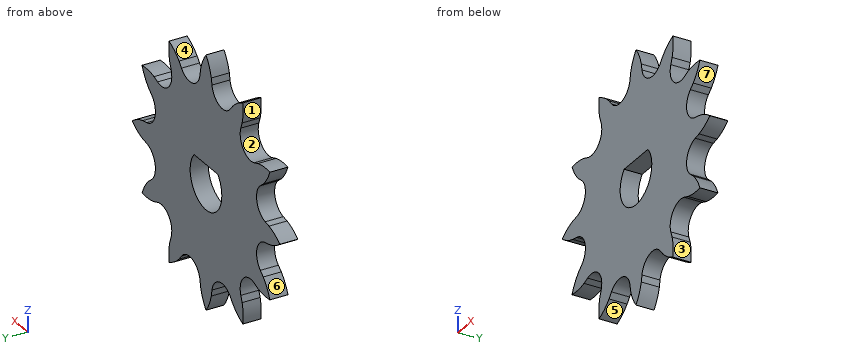
from build123d import *

# Parameters (mm, degrees)
SKETCH1_R           = 10
BOSS_EXTRUDE3_DEPTH = 2
CUT_EXTRUDE4_START  = -2
CUT_EXTRUDE4_DEPTH  = 2
CUT_EXTRUDE5_DEPTH  = 2
CUT_EXTRUDE7_START  = -2
CUT_EXTRUDE7_DEPTH  = 2


with BuildPart() as part:
    # Sketch1 → Boss-Extrude3 (new body)
    # profile 1 of 3: a face of its own
    with BuildSketch(Plane(origin=(0, 0, 0), x_dir=(1, 0, 0), z_dir=(0, 1, 0))):
        with BuildLine():
            ThreePointArc((-2.576546391, 9.66237076), (-3.696714803, 9.688501423), (-4.6270391, 10.312966622))
            Line((-4.6270391, 10.312966622), (-5.089759275, 10.867122458))
            add(Edge.make_bspline(
                [(-5.089759275, 10.867122458), (-6.64901802, 12.325915574), (-6.970753087, 12.141194398)],
                knots=[0, 0, 0, 1, 1, 1], degree=2, weights=[1, 1.687053572, 1]))
            ThreePointArc((-6.970753087, 12.141194398), (-7.014608214, -12.115909855), (14, 0))
            ThreePointArc((14, 0), (9.899494937, 9.899494937), (0, 14))
            add(Edge.make_bspline(
                [(-0.996876474, 11.958521535), (-0.370992408, 14), (0, 14)],
                knots=[0, 0, 0, 1, 1, 1], degree=2, weights=[1, 1.687053572, 1]))
            Line((-0.996876474, 11.958521535), (-1.122240194, 11.247548548))
            ThreePointArc((-1.122240194, 11.247548548), (-1.618115564, 10.242776114), (-2.576546391, 9.66237076))
        make_face()
        with BuildLine():
            ThreePointArc((10, 0), (-6.092394278, -7.9298633), (-2.576546391, 9.66237076))
            ThreePointArc((-2.576546391, 9.66237076), (6.092394278, 7.9298633), (10, 0))
        make_face(mode=Mode.SUBTRACT)
    # profile 2 of 3: a face of its own
    with BuildSketch(Plane(origin=(0, 0, 0), x_dir=(1, 0, 0), z_dir=(0, 1, 0))):
        Circle(SKETCH1_R)
    # profile 3 of 3: a face of its own
    with BuildSketch(Plane(origin=(0, 0, 0), x_dir=(1, 0, 0), z_dir=(0, 1, 0))):
        with BuildLine():
            Line((-5.089759275, 10.867122458), (-4.6270391, 10.312966622))
            ThreePointArc((-4.6270391, 10.312966622), (-3.696714803, 9.688501423), (-2.576546391, 9.66237076))
            ThreePointArc((-2.576546391, 9.66237076), (-1.618115564, 10.242776114), (-1.122240194, 11.247548548))
            Line((-1.122240194, 11.247548548), (-0.996876474, 11.958521535))
            add(Edge.make_bspline(
                [(-0.996876474, 11.958521535), (-0.370992408, 14), (0, 14)],
                knots=[0, 0, 0, 1, 1, 1], degree=2, weights=[1, 1.687053572, 1]))
            ThreePointArc((0, 14), (-3.607164983, 13.527319054), (-6.970753087, 12.141194398))
            add(Edge.make_bspline(
                [(-5.089759275, 10.867122458), (-6.64901802, 12.325915574), (-6.970753087, 12.141194398)],
                knots=[0, 0, 0, 1, 1, 1], degree=2, weights=[1, 1.687053572, 1]))
        make_face()
    extrude(amount=BOSS_EXTRUDE3_DEPTH)

    # Sketch2 → Cut-Extrude4 (cut)
    with BuildSketch(Plane(origin=(0, 2, 0), x_dir=(1, 0, 0), z_dir=(0, 1, 0)).offset(CUT_EXTRUDE4_START)):
        with BuildLine():
            Line((-1.136213035, 11.24381356), (-1.010390736, 11.95738728))
            ThreePointArc((-1.010390736, 11.95738728), (-0.613638742, 13.032335811), (0, 14))
            ThreePointArc((0, 14), (-3.623466631, 13.522961568), (-7, 12.124355653))
            ThreePointArc((-7, 12.124355653), (-5.984741166, 11.593153253), (-5.103669595, 10.860596515))
            Line((-5.103669595, 10.860596515), (-4.637917427, 10.305534696))
            ThreePointArc((-4.637917427, 10.305534696), (-2.588190451, 9.659258263), (-1.136213035, 11.24381356))
        make_face()
    extrude(amount=CUT_EXTRUDE4_DEPTH, mode=Mode.SUBTRACT)

    # Sketch3 → Cut-Extrude5 (cut)
    with BuildSketch(Plane(origin=(0, 2, 0), x_dir=(1, 0, 0), z_dir=(0, 1, 0))):
        with BuildLine():
            Line((-2.25, -1.984313483), (2.25, -1.984313483))
            ThreePointArc((2.25, -1.984313483), (0, 3), (-2.25, -1.984313483))
        make_face()
    extrude(amount=-CUT_EXTRUDE5_DEPTH, mode=Mode.SUBTRACT)

    # Sketch2<5> → Cut-Extrude7 (cut)
    with BuildSketch(Plane(origin=(0, 2, 0), x_dir=(1, 0, 0), z_dir=(0, 1, 0)).offset(CUT_EXTRUDE7_START)):
        with BuildLine():
            ThreePointArc((7, 12.124355653), (3.623466631, 13.522961568), (0, 14))
            ThreePointArc((0, 14), (0.613638742, 13.032335811), (1.010390736, 11.95738728))
            Line((1.010390736, 11.95738728), (1.136213035, 11.24381356))
            ThreePointArc((1.136213035, 11.24381356), (2.588190451, 9.659258263), (4.637917427, 10.305534696))
            Line((4.637917427, 10.305534696), (5.103669595, 10.860596515))
            ThreePointArc((5.103669595, 10.860596515), (5.984741166, 11.593153253), (7, 12.124355653))
        make_face()
        with BuildLine():
            ThreePointArc((12.124355653, 7), (9.899494937, 9.899494937), (7, 12.124355653))
            ThreePointArc((7, 12.124355653), (7.047594644, 10.979514512), (6.853717685, 9.850205779))
            Line((6.853717685, 9.850205779), (6.605896133, 9.169321661))
            ThreePointArc((6.605896133, 9.169321661), (7.071067812, 7.071067812), (9.169321661, 6.605896133))
            Line((9.169321661, 6.605896133), (9.850205779, 6.853717685))
            ThreePointArc((9.850205779, 6.853717685), (10.979514512, 7.047594644), (12.124355653, 7))
        make_face()
        with BuildLine():
            ThreePointArc((14, 0), (13.522961568, 3.623466631), (12.124355653, 7))
            ThreePointArc((12.124355653, 7), (11.593153253, 5.984741166), (10.860596515, 5.103669595))
            Line((10.860596515, 5.103669595), (10.305534696, 4.637917427))
            ThreePointArc((10.305534696, 4.637917427), (9.659258263, 2.588190451), (11.24381356, 1.136213035))
            Line((11.24381356, 1.136213035), (11.95738728, 1.010390736))
            ThreePointArc((11.95738728, 1.010390736), (13.032335811, 0.613638742), (14, 0))
        make_face()
        with BuildLine():
            ThreePointArc((-6.853717685, 9.850205779), (-7.047594644, 10.979514512), (-7, 12.124355653))
            ThreePointArc((-7, 12.124355653), (-9.899494937, 9.899494937), (-12.124355653, 7))
            ThreePointArc((-12.124355653, 7), (-10.979514512, 7.047594644), (-9.850205779, 6.853717685))
            Line((-9.850205779, 6.853717685), (-9.169321661, 6.605896133))
            ThreePointArc((-9.169321661, 6.605896133), (-7.071067812, 7.071067812), (-6.605896133, 9.169321661))
            Line((-6.605896133, 9.169321661), (-6.853717685, 9.850205779))
        make_face()
        with BuildLine():
            ThreePointArc((12.124355653, -7), (13.522961568, -3.623466631), (14, 0))
            ThreePointArc((14, 0), (13.032335811, -0.613638742), (11.95738728, -1.010390736))
            Line((11.95738728, -1.010390736), (11.24381356, -1.136213035))
            ThreePointArc((11.24381356, -1.136213035), (9.659258263, -2.588190451), (10.305534696, -4.637917427))
            Line((10.305534696, -4.637917427), (10.860596515, -5.103669595))
            ThreePointArc((10.860596515, -5.103669595), (11.593153253, -5.984741166), (12.124355653, -7))
        make_face()
        with BuildLine():
            ThreePointArc((-10.860596515, 5.103669595), (-11.593153253, 5.984741166), (-12.124355653, 7))
            ThreePointArc((-12.124355653, 7), (-13.522961568, 3.623466631), (-14, 0))
            ThreePointArc((-14, 0), (-13.032335811, 0.613638742), (-11.95738728, 1.010390736))
            Line((-11.95738728, 1.010390736), (-11.24381356, 1.136213035))
            ThreePointArc((-11.24381356, 1.136213035), (-9.659258263, 2.588190451), (-10.305534696, 4.637917427))
            Line((-10.305534696, 4.637917427), (-10.860596515, 5.103669595))
        make_face()
        with BuildLine():
            ThreePointArc((7, -12.124355653), (9.899494937, -9.899494937), (12.124355653, -7))
            ThreePointArc((12.124355653, -7), (10.979514512, -7.047594644), (9.850205779, -6.853717685))
            Line((9.850205779, -6.853717685), (9.169321661, -6.605896133))
            ThreePointArc((9.169321661, -6.605896133), (7.071067812, -7.071067812), (6.605896133, -9.169321661))
            Line((6.605896133, -9.169321661), (6.853717685, -9.850205779))
            ThreePointArc((6.853717685, -9.850205779), (7.047594644, -10.979514512), (7, -12.124355653))
        make_face()
        with BuildLine():
            ThreePointArc((-11.95738728, -1.010390736), (-13.032335811, -0.613638742), (-14, 0))
            ThreePointArc((-14, 0), (-13.522961568, -3.623466631), (-12.124355653, -7))
            ThreePointArc((-12.124355653, -7), (-11.593153253, -5.984741166), (-10.860596515, -5.103669595))
            Line((-10.860596515, -5.103669595), (-10.305534696, -4.637917427))
            ThreePointArc((-10.305534696, -4.637917427), (-9.659258263, -2.588190451), (-11.24381356, -1.136213035))
            Line((-11.24381356, -1.136213035), (-11.95738728, -1.010390736))
        make_face()
        with BuildLine():
            ThreePointArc((0, -14), (3.623466631, -13.522961568), (7, -12.124355653))
            ThreePointArc((7, -12.124355653), (5.984741166, -11.593153253), (5.103669595, -10.860596515))
            Line((5.103669595, -10.860596515), (4.637917427, -10.305534696))
            ThreePointArc((4.637917427, -10.305534696), (2.588190451, -9.659258263), (1.136213035, -11.24381356))
            Line((1.136213035, -11.24381356), (1.010390736, -11.95738728))
            ThreePointArc((1.010390736, -11.95738728), (0.613638742, -13.032335811), (0, -14))
        make_face()
        with BuildLine():
            ThreePointArc((-9.850205779, -6.853717685), (-10.979514512, -7.047594644), (-12.124355653, -7))
            ThreePointArc((-12.124355653, -7), (-9.899494937, -9.899494937), (-7, -12.124355653))
            ThreePointArc((-7, -12.124355653), (-7.047594644, -10.979514512), (-6.853717685, -9.850205779))
            Line((-6.853717685, -9.850205779), (-6.605896133, -9.169321661))
            ThreePointArc((-6.605896133, -9.169321661), (-7.071067812, -7.071067812), (-9.169321661, -6.605896133))
            Line((-9.169321661, -6.605896133), (-9.850205779, -6.853717685))
        make_face()
        with BuildLine():
            ThreePointArc((-7, -12.124355653), (-3.623466631, -13.522961568), (0, -14))
            ThreePointArc((0, -14), (-0.613638742, -13.032335811), (-1.010390736, -11.95738728))
            Line((-1.010390736, -11.95738728), (-1.136213035, -11.24381356))
            ThreePointArc((-1.136213035, -11.24381356), (-2.588190451, -9.659258263), (-4.637917427, -10.305534696))
            Line((-4.637917427, -10.305534696), (-5.103669595, -10.860596515))
            ThreePointArc((-5.103669595, -10.860596515), (-5.984741166, -11.593153253), (-7, -12.124355653))
        make_face()
    extrude(amount=CUT_EXTRUDE7_DEPTH, mode=Mode.SUBTRACT)


solid = part.part
Source: CAD feature listing. Evaluate the final solid. Frame: model axes, mm. Face numbers are marked on the shaded views. A direction names the side the tool comes from. Give positions to 0.01 mm unless a question says otherwise; leave off trailing zeros. Write each loop counter-clockwise with the first axis right and the second up, starting at its lowest first coordinate (ties: lowest second). Pieces come first, ordered by that corner, then holes. Notation, with made-up numbers: M -38.75,-26 L -5.75,-26 A33 ccw -5.75,3 Z; hole C 65.25,24.25 d2. An arc over 180 degrees is marked long. Answer as a JSON object with one key per item and string values.
Q1. Ray query, line 1 along X through (y, z) = (0.8, 9.75); line 2 along X through (y, z) = (0.6, -10.75); line 3 along Z through (x, y) = (-2.5, 1.2). Return the intervals inside material, ascending.
Geometry check:
{"line 1": "x = -6.82 to -3.89, -2.32 to 2.32, 3.89 to 6.82", "line 2": "x = -7.03 to -5.01, -1.29 to 1.29, 5.01 to 7.03", "line 3": "z = -9.69 to -1.66, 1.66 to 9.69"}
Q2. Access query for the marked faces 5, 6 and 7. Directions: +Z, -Z, +X, -X, +Y, -Y. A direction counts if a zero-diameter tool reaches every point of the face in a straight line with its end or side. Return the directions, or none.
Geometry check:
{"face 5": "-Z, +Y, -Y", "face 6": "-X, +Y, -Y", "face 7": "+X, +Y, -Y"}
Q3. Cut plane B-B, the plane z = 3. Return the cut outline in (x, y), then the cut area to 3 significant figures.
Geometry check:
{"outline": "M -9.59,0 L 9.59,0 L 9.59,2 L -9.59,2 Z", "area": "38.4 mm^2"}
Q4. Cut plane A-A, the plane x = 4. Return the cut outline in (y, z).
Geometry check:
{"outline": "M 0,-9.8 L 2,-9.8 L 2,9.8 L 0,9.8 Z"}
Q5. Mould query, pull axis X, two halves, no side actions, for the marked faces 1, 2, 3 and 4. Classes: +X half, -X half, draft (parallel to the pull), parting line (faces both ways), or undercut.
Geometry check:
{"face 1": "-X half", "face 2": "undercut", "face 3": "+X half", "face 4": "undercut"}
